CAD build for the part. Positions are in the model's coordinates, mm. Give positions to 0.01 mm unless a question says otherwise; leave off trailing zeros. Write each loop counter-clockwise with the first axis right and the second up, starting at its lowest first coordinate (ties: lowest second). Pieces come first, ordered by that corner, then holes. Notation, with made-up numbers: (-20, -10.5) - (27, -10.5) arc R35 cw to (27, 28.5) - close; hole circle Ø3 at (67, 40). An arc over 180 degrees is marked (long way). Put each result on its own line as item: value. Start each with the question number.
1. Cut at B-B on z = -1.4. List the corners of the cut face in (x, y).
2. Cut at A-A on x = 0. List the corners of the cut face in (y, z) (3 decimals), and give its area (3 significant figures).
3. Drop flat-ended pins along their axis: pin 1 (1 mm diameter, centred on y = -2, z = -2.5, fed in from -X); pin 2 (3 mm diameter, centred on x = 0, y = 0, fed in from +Z); pin 3 (1.5 mm diameter, centred on y = 3, z = -3.5, fed in from -X); pin 4 (5.5 mm diameter, centred on x = 1, y = 0.5, fed in from +Z). Give the stop position or say it passes through.
4. Mould opens along Y. For faces 1 (the flat face through (-2.4, 0.1, -4.572)), 2 (the flat face through (-2.4, -0.1, -4.318)), 3 (the cylindrical face through (-6.695, -1.487, -2.029)) say: +Y half, -Y half, draft (parallel to the pull), parting line (faces both ways), or undercut.
5. Wall check: line 1 (X direction, y = 0, z = -2); line 2 (Y direction, x = 0.25, z = -3.2); line 3 (Z direction, x = -3, y = 3.75). Give the ranges that are in metal, low to high.
from build123d import *


with BuildPart() as part:
    # Sketch1 → Revolve1 (revolve)
    with BuildSketch(Plane(origin=(0, 0, 0), x_dir=(0, 0, -1), z_dir=(1, 0, 0))):
        with BuildLine():
            Line((0, 8.001), (0, 7.747))
            ThreePointArc((0, 7.747), (0.21198872, 7.056541514), (0.774908178, 6.604))
            Line((0.774908178, 6.604), (3.31799946, 6.604))
            ThreePointArc((3.31799946, 6.604), (4.025106623, 6.311106623), (4.318, 5.60399946))
            Line((4.318, 5.60399946), (4.318, 1.905))
            Line((4.318, 1.905), (4.572, 1.905))
            Line((4.572, 1.905), (4.572, 5.60399946))
            ThreePointArc((4.572, 5.60399946), (4.204711745, 6.490711745), (3.31799946, 6.858))
            Line((3.31799946, 6.858), (0.774908178, 6.858))
            ThreePointArc((0.774908178, 6.858), (0.393818958, 7.231814031), (0.254, 7.747))
            Line((0.254, 7.747), (0.254, 8.001))
            Line((0.254, 8.001), (0, 8.001))
        make_face()
    revolve(axis=Axis((0, 0, 11.444404328), (0, 0, -1)))


solid = part.part
Report:
1. outline: circle Ø13.72 at (0, 0); hole circle Ø13.21 at (0, 0)
2. outline: (-8.001, -0.254) - (-7.747, -0.254) arc R1.019 cw to (-6.858, -0.775) - (-6.858, -3.318) arc R1.254 ccw to (-5.604, -4.572) - (-1.905, -4.572) - (-1.905, -4.318) - (-5.604, -4.318) arc R1 cw to (-6.604, -3.318) - (-6.604, -0.775) arc R1.23 ccw to (-7.747, 0) - (-8.001, 0) - close; (1.905, -4.572) - (5.604, -4.572) arc R1.254 ccw to (6.858, -3.318) - (6.858, -0.775) arc R1.019 cw to (7.747, -0.254) - (8.001, -0.254) - (8.001, 0) - (7.747, 0) arc R1.23 ccw to (6.604, -0.775) - (6.604, -3.318) arc R1 cw to (5.604, -4.318) - (1.905, -4.318) - close
2. area: 4.82 mm²
3. pin 1: stops at x = -6.69
3. pin 2: passes through
3. pin 3: stops at x = -6.47
3. pin 4: stops at z = -4.32
4. face 1: draft
4. face 2: undercut
4. face 3: parting line
5. line 1: x = -6.86 to -6.6, 6.6 to 6.86
5. line 2: y = -6.85 to -6.6, 6.6 to 6.85
5. line 3: z = -4.57 to -4.32
